Geometry check sheet. Reference: the model listing, model coordinates, mm. A direction names the side the tool comes from. Round coordinates to 2 decimals unless told otherwise and drop trailing zeros. Loops run counter-clockwise (first coordinate to the right, second up) from the corner with the lowest first, then second, coordinate; pieces in that order, holes last. Notation, with made-up numbers: (86.25, -40) -> (126.25, -40) arc R21 cw to (126.25, -13) -> close; hole circle Ø2 at (34, -4). An arc over 180 degrees is marked (long way). Use a Markdown table: item, result. Add a question column.
Q1. Release check for a two-part mould opening along Z. For faces 6 (the face through (-24, -7, 7.5)), 7 (the face through (-9, -1, -15.5)), 8 (the face through (15.5, -1, 0)), 9 (the face through (-23, -6, 8.5)) record: released by +Z, released by -Z, zero draft, split by the parting line, or undercut.
Q2. Material ranges on L1, parallel to Z at x = 0, y = -1.2; L2, parallel to X at y = -4.5, z = -7; L3, parallel to X at y = -2.75, z = -7.5, recorded low to high.
Q3. Sectioned sample at B-B, the plane x = 0. Enter the section's corners in (y, z), then the cut area to 3 significant figures.
Q4. Sectioned sample at C-C, the plane y = -1.75. Enter the section's corners in (x, z), then the cut area to 3 significant figures.
Q5. Gauge pin test, flat ends, axial feed: P1, Ø10, axis at x = 0.5, z = 8, coming from the -Y side; P2, Ø4, axis at x = -28, y = -5, coming from the +Z side; P3, Ø2, axis at y = -7.5, z = 6.5, coming from the +X side. Record the tip position at first contact, or that the pin passes through.
Q6. Sectioned sample at D-D, the plane x = -14.5. Enter the section's corners in (y, z), then the cut area to 3 significant figures.
Q7. Sectioned sample at A-A, the plane z = 10. Enter the section's corners in (x, y), then the cut area to 4 significant figures.
Q8. Set-up check for faces 1 (the face through (-22, -10, -8)), 2 (the face through (-9, -1, 15.5)), 3 (the face through (-14, -6, 0)), 4 (the face through (-24, -4, 0)), 5 (the face through (-23, -6, -8.5)): record each of +Z, -Z, +X, -X, +Y, -Y from which the full face is reachable in a straight line by a thin tool's end or side.
Autodesk Inventor part; units mm, degrees
ref_plane "YZ Plane" through (0, 0, 0) normal (1, 0, 0) x (0, 1, 0)
ref_plane "XZ Plane" through (0, 0, 0) normal (0, 1, 0) x (-1, 0, 0)
ref_plane "XY Plane" through (0, 0, 0) normal (0, 0, 1) x (1, 0, 0)
sketch "Sketch1" plane through (0, 0, 0) normal (0, 1, 0) x (-1, 0, 0)
  circle A0 centre (0, 0) radius 12.5
  line L0 (0, -12.5) -> (30, -12.5) construction
  line L1 (0, 12.5) -> (30, 12.5) construction
  line L2 (30, 12.5) -> (30, -12.5) construction
  line L3 (0, -12.5) -> (16, -12.5) construction
  line L4 (0, 12.5) -> (16, 12.5) construction
  line L5 (16, 12.5) -> (16, -12.5) construction
  line L6 (30, 12.5) -> (30, 8.5) construction
  line L7 (30, -12.5) -> (30, -8.5) construction
  line L8 (0, -12.5) -> (0, -15.5) construction
  line L9 (0, 12.5) -> (0, 15.5) construction
  line L10 (30, -1.5) -> (33, -1.5) construction
  line L11 (-12.5, 0) -> (-15.5, 0) construction
  line L12 (33, -1.5) -> (33, -15.5)
  line L13 (33, -15.5) -> (0, -15.5)
  line L14 (33, -1.5) -> (33, 15.5)
  line L15 (33, 15.5) -> (0, 15.5)
  line L16 (0, 15.5) -> (-15.5, 15.5)
  line L17 (-15.5, 0) -> (-15.5, 15.5)
  line L18 (0, -15.5) -> (-15.5, -15.5)
  line L19 (-15.5, -15.5) -> (-15.5, 0)
  line L20 (0, 12.5) -> (14, 12.5) construction
  line L21 (0, -12.5) -> (14, -12.5) construction
  line L22 (14, 12.5) -> (14, -12.5) construction
  line L23 (33, 8.5) -> (33, 11.5) construction
  line L24 (33, -8.5) -> (33, -9.5) construction
  line L25 (14, -11.5) -> (14, -6.5) construction
  line L26 (14, 10.5) -> (14, 5.5) construction
  line L27 (0, -12.5) -> (15, -12.5) construction
  line L28 (0, 12.5) -> (15, 12.5) construction
  line L29 (15, 12.5) -> (15, -12.5) construction
  line L30 (14, -11.5) -> (14, -6.5) construction
  line L31 (14, -12.5) -> (14, -7.5) construction
  line L32 (14, 12.5) -> (14, 7.5) construction
  line L33 (14, 7.5) -> (30, 7.5) construction
  line L34 (14, -7.5) -> (30, -7.5) construction
  line L35 (16, -7.5) -> (16, -8.5) construction
  line L36 (16, 7.5) -> (16, 8.5) construction
  line L37 (16, 7.5) -> (16, 6.5) construction
  line L38 (16, -7.5) -> (16, -6.5) construction
  line L39 (30, -8.5) -> (14, -8.5) construction
  line L40 (30, 8.5) -> (14, 8.5) construction
  line L41 (14, -8.5) -> (33, -8.5)
  line L42 (14, 8.5) -> (33, 8.5)
  line L43 (33, 7.5) -> (15, 7.5)
  line L44 (15, 7.5) -> (15, -7.5)
  line L45 (15, -7.5) -> (33, -7.5)
  line L46 (14, -8.5) -> (14, 8.5)
  line L47 (33, -8.5) -> (33, 7.5)
  dimension "d0" = 25
  dimension "d1" = 30
  dimension "d2" = 30
  dimension "d3" = 16
  dimension "d4" = 16
  dimension "d5" = 4
  dimension "d6" = 4
  dimension "d7" = 3
  dimension "d8" = 3
  dimension "d9" = 3
  dimension "d10" = 3
  dimension "d16" = 14
  dimension "d17" = 14
  dimension "d26" = 15
  dimension "d27" = 15
  dimension "d29" = 5
  dimension "d30" = 5
  dimension "d31" = 1
  dimension "d32" = 1
  dimension "d33" = 1
  dimension "d34" = 1
extrude "Extrusion5" add sketch "Sketch1" against normal blind 2.5 contours L12 L13 L18 L19 L17 L16 L15 L14 L42 L46 L41
extrude "Extrusion6" add sketch "Sketch1" against normal blind 10 contours L12 L41 L46 L42 L14 L43 L44 L45
extrude "Extrusion7" add sketch "Sketch1" against normal blind 4 contours L12 L45 L44 L43 L14
properties part number "joystick_test_v2_3DPrint"
Values:
| question | item | result |
|---|---|---|
| 1 | face 6 | undercut |
| 1 | face 7 | released by -Z |
| 1 | face 8 | zero draft |
| 1 | face 9 | released by +Z |
| 2 | L1 | -15.5 to -12.5, 12.5 to 15.5 |
| 2 | L2 | -15 to -14 |
| 2 | L3 | -33 to -14 |
| 3 | outline | (-2.5, -15.5) -> (0, -15.5) -> (0, -12.5) -> (-2.5, -12.5) -> close; (-2.5, 12.5) -> (0, 12.5) -> (0, 15.5) -> (-2.5, 15.5) -> close |
| 3 | area | 15.0 mm^2 |
| 4 | outline | (-33, -15.5) -> (15.5, -15.5) -> (15.5, 15.5) -> (-33, 15.5) -> close; hole circle Ø25 at (0, 0) |
| 4 | area | 1,010 mm^2 |
| 5 | P1 | y = -2.5 |
| 5 | P2 | z = 8.5 |
| 5 | P3 | x = -14 |
| 6 | outline | (-10, -8.5) -> (-2.5, -8.5) -> (-2.5, -15.5) -> (0, -15.5) -> (0, 15.5) -> (-2.5, 15.5) -> (-2.5, 8.5) -> (-10, 8.5) -> close |
| 6 | area | 205 mm^2 |
| 7 | outline | (-33, -2.5) -> (-7.5, -2.5) -> (-7.5, 0) -> (-33, 0) -> close; (7.5, -2.5) -> (15.5, -2.5) -> (15.5, 0) -> (7.5, 0) -> close |
| 7 | area | 83.75 mm^2 |
| 8 | face 1 | +Z, -Z, +X, -X, -Y |
| 8 | face 2 | +Z, +X, -X, +Y, -Y |
| 8 | face 3 | +Z, -Z, +X, -Y |
| 8 | face 4 | -X, -Y |
| 8 | face 5 | -Z, +X, -X, -Y |
